The model under review builds one solid part; all positions refer to its coordinate system, in mm. Face numbers are marked on the shaded views. A direction names the side the tool comes from. Round coordinates to 2 decimals unless told otherwise and drop trailing zeros. Loops run counter-clockwise (first coordinate to the right, second up) from the corner with the lowest first, then second, coordinate; pieces in that order, holes last. Notation, with made-up numbers: M 88,-32.75 L 138,-32.75 A22 ccw 138,-22.75 Z; hole C 32.25,55.25 d9. An arc over 180 degrees is marked long. Return JSON: item names as keys, results as strings. Group by question number.
Q1. To check wall thickness, follow line 1 along X through (y, z) = (1.5, -3.25); line 2 along Y through (x, z) = (-3.3, -3.3); line 3 along Y through (x, z) = (3.3, 4.75). State the ranges of each line that lie inside material, in increasing order.
Q2. Consider section D-D (y = 0). State the section outline as (x, z) points, and give its area (3 significant figures).
Q3. Consider section A-A (x = 8). State the section outline as (y, z) points, and give its area (3 significant figures).
Q4. Consider section C-C (z = 2). State the section outline as (x, y) points, and give its area (3 significant figures).
Q5. Draft analysis for pull direction X (two halves, no side actions). For the marked faces 1, 2 and 3, state which applies: pulls with the +X half, pulls with the -X half, needs draft (parallel to the pull), parting line crosses it, or undercut.
Q6. Consider section B-B (z = -1.5). State the section outline as (x, y) points, and give its area (3 significant figures).
Q7. Clearance check with flat-ended pins moving along their axes: pin 1 Ø2 at (y, z) = (1, -3.5) entering from +X; pin 2 Ø3 at (x, z) = (-2.5, 3) entering from -Y; pin 3 Ø3 at (x, y) = (-8, 0) entering from -Z. State where each tip first meets the part, or that it passes through.
Q8. For the marked faces 4, 5, 6 and 7, list the 3-axis set-ups (+Z, -Z, +X, -X, +Y, -Y) from which the entire face can be reached by the end or side of a thin tool; tool diameter is ignored.
from build123d import *

# Parameters (mm, degrees)
SKETCH_2_W      = 10
SKETCH_2_H      = 6.5
SKETCH_2_R      = 0.5
EXTRUDE_1_DEPTH = 6.7
SKETCH_4_W      = 20
SKETCH_4_H      = 8.6
SKETCH_4_R      = 1
EXTRUDE_2_DEPTH = 2
EXTRUDE_START   = 2
SKETCH_7_W      = 10.8
SKETCH_7_H      = 6.8
SKETCH_7_R      = 0.5
EXTRUDE_3_DEPTH = 2
FILLET_1_R      = 1
FILLET_2_R      = 1
FILLET_4_R      = 0.5


with BuildPart() as part:
    # 草图2 → 凸台-拉伸1 (new body)
    with BuildSketch(Plane.XY):
        Rectangle(SKETCH_2_W, SKETCH_2_H)
        with Locations((-3.3, 1.5)):
            Circle(SKETCH_2_R, mode=Mode.SUBTRACT)
        with Locations((0, 1.5)):
            Circle(SKETCH_2_R, mode=Mode.SUBTRACT)
        with Locations((3.3, 1.5)):
            Circle(SKETCH_2_R, mode=Mode.SUBTRACT)
        with Locations((0, -1.5)):
            Circle(SKETCH_2_R, mode=Mode.SUBTRACT)
        with Locations((3.3, -1.5)):
            Circle(SKETCH_2_R, mode=Mode.SUBTRACT)
        with Locations((-3.3, -1.5)):
            Circle(SKETCH_2_R, mode=Mode.SUBTRACT)
    extrude(amount=EXTRUDE_1_DEPTH)

    # 草图4 → 凸台-拉伸2 (add)
    with BuildSketch(Plane.XY):
        Rectangle(SKETCH_4_W, SKETCH_4_H)
        with Locations((-8, 0)):
            Circle(SKETCH_4_R, mode=Mode.SUBTRACT)
        with Locations(Location((8, 0, 0), (0, 0, 180))):
            Circle(SKETCH_4_R, mode=Mode.SUBTRACT)
    extrude(amount=-EXTRUDE_2_DEPTH)

    # 草图7 → 凸台-拉伸3 (add)
    with BuildSketch(Plane(origin=(0, 0, -2), x_dir=(-1, 0, 0), z_dir=(0, 0, -1)).offset(EXTRUDE_START)):
        Rectangle(SKETCH_7_W, SKETCH_7_H)
        with Locations(Location((-3.3, 1.5, 0), (0, 0, 180))):
            Circle(SKETCH_7_R, mode=Mode.SUBTRACT)
        with Locations(Location((0, 1.5, 0), (0, 0, 180))):
            Circle(SKETCH_7_R, mode=Mode.SUBTRACT)
        with Locations(Location((3.3, 1.5, 0), (0, 0, 180))):
            Circle(SKETCH_7_R, mode=Mode.SUBTRACT)
        with Locations(Location((0, -1.5, 0), (0, 0, 180))):
            Circle(SKETCH_7_R, mode=Mode.SUBTRACT)
        with Locations(Location((3.3, -1.5, 0), (0, 0, 180))):
            Circle(SKETCH_7_R, mode=Mode.SUBTRACT)
        with Locations(Location((-3.3, -1.5, 0), (0, 0, 180))):
            Circle(SKETCH_7_R, mode=Mode.SUBTRACT)
    extrude(amount=-EXTRUDE_3_DEPTH)

    # 圆角1
    fillet_1_edges = [part.edges().sort_by_distance(p)[0] for p in [
        (10, 4.3, -1),
        (10, -4.3, -1),
        (-10, -4.3, -1),
        (-10, 4.3, -1),
    ]]
    fillet(fillet_1_edges, radius=FILLET_1_R)

    # 圆角2
    fillet_2_edges = [part.edges().sort_by_distance(p)[0] for p in [
        (5, -3.25, 3.35),
        (5, 3.25, 3.35),
        (5.4, 3.4, -3),
        (5.4, -3.4, -3),
    ]]
    fillet(fillet_2_edges, radius=FILLET_2_R)

    # 圆角4
    fillet_4_edges = [part.edges().sort_by_distance(p)[0] for p in [
        (-5, 0, 6.7),
        (5, 0, 6.7),
        (-0.5, 3.25, 6.7),
        (4.707106781, 2.957106781, 6.7),
        (4.707106781, -2.957106781, 6.7),
        (-0.5, -3.25, 6.7),
    ]]
    fillet(fillet_4_edges, radius=FILLET_4_R)


solid = part.part
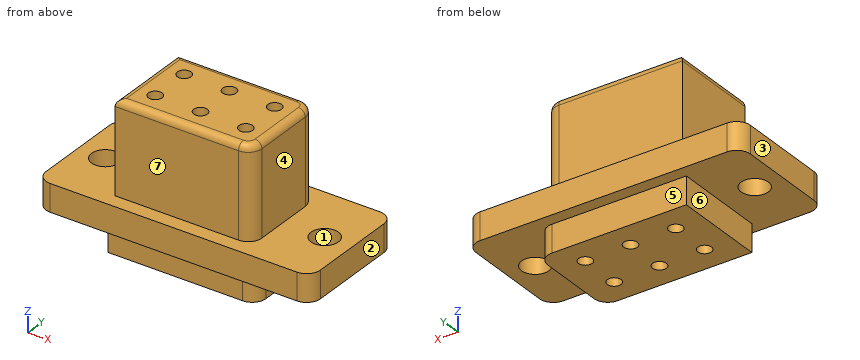
Values:
{
 "1": {"line 1": "x = -5.4 to -3.8, -2.8 to -0.5, 0.5 to 2.8, 3.8 to 5.4", "line 2": "y = -3.4 to -2, -1 to 1, 2 to 3.4", "line 3": "y = -3.25 to -2, -1 to 1, 2 to 3.25"},
 "2": {"outline": "M -10,-2 L -9,-2 L -9,0 L -10,0 Z; M -7,-2 L -5.4,-2 L -5.4,-4 L 5.4,-4 L 5.4,-2 L 7,-2 L 7,0 L 5,0 L 5,6.2 A0.5 ccw 4.5,6.7 L -4.5,6.7 A0.5 ccw -5,6.2 L -5,0 L -7,0 Z; M 9,-2 L 10,-2 L 10,0 L 9,0 Z", "area": "120 mm2"},
 "3": {"outline": "M -4.3,-2 L -1,-2 L -1,0 L -4.3,0 Z; M 1,-2 L 4.3,-2 L 4.3,0 L 1,0 Z", "area": "13.2 mm2"},
 "4": {"outline": "M -5,-3.25 L 4,-3.25 A1 ccw 5,-2.25 L 5,2.25 A1 ccw 4,3.25 L -5,3.25 Z; hole C -3.3,-1.5 d1; hole C -3.3,1.5 d1; hole C 0,-1.5 d1; hole C 0,1.5 d1; hole C 3.3,-1.5 d1; hole C 3.3,1.5 d1", "area": "59.9 mm2"},
 "5": {"face 1": "undercut", "face 2": "pulls with the +X half", "face 3": "pulls with the -X half"},
 "6": {"outline": "M -10,-3.3 A1 ccw -9,-4.3 L 9,-4.3 A1 ccw 10,-3.3 L 10,3.3 A1 ccw 9,4.3 L -9,4.3 A1 ccw -10,3.3 Z; hole C -8,0 d2; hole C 8,0 d2", "area": "165 mm2"},
 "7": {"pin 1": "stops at x = 5.4", "pin 2": "stops at y = -3.25", "pin 3": "stops at z = -2"},
 "8": {"face 4": "+Z, +X, +Y, -Y", "face 5": "-Z, +X, -X, +Y", "face 6": "-Z, -X, +Y, -Y", "face 7": "+Z, +X, -X, -Y"}
}
